```python
from build123d import *

# Parameters (mm, degrees)
SKETCH001_W     = 178
SKETCH001_H     = 55
SKETCH001_R     = 2.5
SKETCH001_R_2   = 8
SKETCH001_R_3   = 12.004096
PAD_DEPTH       = 1
SKETCH004_R     = 1.3
POCKET_DEPTH    = 9
SKETCH003_R     = 4
PAD001_DEPTH    = 8
SKETCH006_W     = 178
SKETCH006_H     = 55
SKETCH006_R     = 2.5
SKETCH006_R_2   = 8
SKETCH006_R_3   = 12.004096
PAD002_DEPTH    = 4
SKETCH_R        = 1.3
POCKET001_DEPTH = 13.001
SKETCH007_R     = 1.3
POCKET002_DEPTH = 5.001
FILLET_R        = 2


with BuildPart() as part:
    # Sketch001 → Pad (new body)
    with BuildSketch(Plane.XY):
        with Locations((-27.95005, 210.084131)):
            Rectangle(SKETCH001_W, SKETCH001_H)
        with Locations((5.54995, 200.560838)):
            Circle(SKETCH001_R, mode=Mode.SUBTRACT)
        with Locations((-105.249172, 192.692063)):
            Circle(SKETCH001_R_2, mode=Mode.SUBTRACT)
        with Locations((44.750828, 192.692063)):
            Circle(SKETCH001_R_2, mode=Mode.SUBTRACT)
        with Locations((42.270485, 220.407623)):
            Circle(SKETCH001_R_3, mode=Mode.SUBTRACT)
        with BuildLine():
            ThreePointArc((25.54995, 206.028969), (20.061493, 220.835101), (5.54995, 227.060838))
            Line((-1.19441, 227.060838), (5.54995, 227.060838))
            Line((-9.694456, 218.560838), (-1.19441, 227.060838))
            Line((-113.95005, 218.561117), (-9.694456, 218.560838))
            Line((-113.95005, 218.561117), (-113.95005, 209.560838))
            Line((-113.95005, 209.560838), (-9.618024, 209.560838))
            Line((-9.618024, 209.560838), (5.54995, 209.560838))
            Line((5.54995, 209.560838), (10.697892, 204.412896))
            Line((10.697892, 189.560838), (10.697892, 204.412896))
            ThreePointArc((10.697892, 189.560838), (21.441031, 194.803313), (25.54995, 206.028969))
        make_face(mode=Mode.SUBTRACT)
        with BuildLine():
            ThreePointArc((-74.793427, 198.14003), (-81.282837, 191.65062), (-74.793427, 185.16121))
            Line((-74.793427, 185.16121), (-26.440948, 185.16121))
            ThreePointArc((-26.440948, 185.16121), (-19.951538, 191.65062), (-26.440948, 198.14003))
            Line((-74.793427, 198.14003), (-26.440948, 198.14003))
        make_face(mode=Mode.SUBTRACT)
        with BuildLine():
            ThreePointArc((-94.612823, 233.364261), (-96.6561, 231.320984), (-94.612823, 229.277707))
            Line((-94.612823, 229.277707), (25.728859, 229.277707))
            ThreePointArc((25.728859, 229.277707), (27.772136, 231.320984), (25.728859, 233.364261))
            Line((-94.612823, 233.364261), (25.728859, 233.364261))
        make_face(mode=Mode.SUBTRACT)
    extrude(amount=PAD_DEPTH)

    # Sketch004 → Pocket (cut)
    with BuildSketch(Plane.XY.offset(10)):
        with Locations((-84.917816, 197.526398)):
            Circle(SKETCH004_R)
        with Locations((-104.937256, 231.505722)):
            Circle(SKETCH004_R)
    extrude(amount=-POCKET_DEPTH, mode=Mode.SUBTRACT)

    # Sketch003 (on Face28 of Pad) → Pad001 (join)
    with BuildSketch(Plane.XY.offset(1)):
        with Locations((-84.943253, 198.501221)):
            Circle(SKETCH003_R)
        with Locations((-104.954079, 231.041534)):
            Circle(SKETCH003_R)
    extrude(amount=PAD001_DEPTH)

    # Sketch006 → Pad002 (join)
    with BuildSketch(Plane.XY):
        with Locations((-27.95005, 210.084131)):
            Rectangle(SKETCH006_W, SKETCH006_H)
        with Locations((5.54995, 200.560838)):
            Circle(SKETCH006_R, mode=Mode.SUBTRACT)
        with Locations((-105.249172, 192.692063)):
            Circle(SKETCH006_R_2, mode=Mode.SUBTRACT)
        with Locations((44.750828, 192.692063)):
            Circle(SKETCH006_R_2, mode=Mode.SUBTRACT)
        with Locations((42.270485, 220.407623)):
            Circle(SKETCH006_R_3, mode=Mode.SUBTRACT)
        with BuildLine():
            ThreePointArc((-74.793427, 198.14003), (-81.282837, 191.65062), (-74.793427, 185.16121))
            Line((-74.793427, 185.16121), (-26.440948, 185.16121))
            ThreePointArc((-26.440948, 185.16121), (-19.951538, 191.65062), (-26.440948, 198.14003))
            Line((-74.793427, 198.14003), (-26.440948, 198.14003))
        make_face(mode=Mode.SUBTRACT)
        with BuildLine():
            ThreePointArc((-94.612823, 233.364261), (-96.6561, 231.320984), (-94.612823, 229.277707))
            Line((-94.612823, 229.277707), (25.728859, 229.277707))
            ThreePointArc((25.728859, 229.277707), (27.772136, 231.320984), (25.728859, 233.364261))
            Line((-94.612823, 233.364261), (25.728859, 233.364261))
        make_face(mode=Mode.SUBTRACT)
    extrude(amount=-PAD002_DEPTH)

    # Sketch (on Face48 of Pad002) → Pocket001 (cut, through all)
    with BuildSketch(Plane.XY.offset(9)):
        with Locations((-84.945648, 198.486725)):
            Circle(SKETCH_R)
        with Locations((-104.952744, 231.032135)):
            Circle(SKETCH_R)
    extrude(amount=-POCKET001_DEPTH, mode=Mode.SUBTRACT)

    # Sketch007 → Pocket002 (cut, through all)
    with BuildSketch(Plane.XY.offset(1)):
        with Locations((44.774215, 204.16173)):
            Circle(SKETCH007_R)
        with Locations((34.814923, 186.91173)):
            Circle(SKETCH007_R)
        with Locations((54.733507, 186.91173)):
            Circle(SKETCH007_R)
        with Locations((-107.25934, 203.941744)):
            Circle(SKETCH007_R)
        with Locations((-114.071897, 185.224398)):
            Circle(SKETCH007_R)
        with Locations((-94.455921, 188.683224)):
            Circle(SKETCH007_R)
    extrude(amount=-POCKET002_DEPTH, mode=Mode.SUBTRACT)

    # Fillet
    fillet_edges = [part.edges().sort_by_distance(p)[0] for p in [
        (-116.95005, 237.584131, -2),
        (-116.95005, 237.584131, 0.5),
        (61.04995, 237.584131, -2),
        (61.04995, 237.584131, 0.5),
        (61.04995, 182.584131, -2),
        (61.04995, 182.584131, 0.5),
        (-116.95005, 182.584131, -2),
        (-116.95005, 182.584131, 0.5),
    ]]
    fillet(fillet_edges, radius=FILLET_R)


solid = part.part
```
Geometry check sheet. Reference: the model listing, model coordinates, mm. A direction names the side the tool comes from. Round coordinates to 2 decimals unless told otherwise and drop trailing zeros. Order: outer loops, then holes, each group sorted by start corner. A loop starts at its lowest first (then second) coordinate and runs counter-clockwise, first axis right, second up. Notation, with made-up numbers: (-33.75, 30) - (14.25, 30) arc R17 cw to (14.25, 36) - close; hole circle Ø5 at (-26.75, -11). An arc over 180 degrees is marked (long way). Use a Markdown table: item, result. Add a question column.
1) Gauge pin test, flat ends, axial feed: P1, Ø3, axis at y = 199.5, z = 3.5, coming from the -X side; P2, Ø4, axis at x = -84.95, y = 198.49, coming from the -Z side; P3, Ø1, axis at y = 200, z = 2.5, coming from the +X side; P4, Ø8, axis at x = -72, y = 226, coming from the +Z side. Record the tip position at first contact, or that the pin passes through.
2) Set-up check for faces 4 (the flat face through (-29, 210, -4)), 5 (the cylindrical face through (-85.81, 194.596, 4.944)): record each of +Z, -Z, +X, -X, +Y, -Y from which the full face is reachable in a straight line by a thin tool's end or side.
3) Section check B-B (y = 217). Record the cut outline in (x, z), then the cut area to 3 significant figures.
4) Section check A-A (x = -4). Record the cut outline in (y, z).
5) Section check D-D (z = -2.5). Count the separate pieces of the cut face and the enclosed holes in it, then the cut area to 3 significant figures.
6) Mould release check, pull along X, two halves, no side actions. Record for faces 1 (the flat face through (61.05, 210, -1)), 2 (the cylindrical face through (20.217, 220.67, 0.493)), 3 (the flat face through (-29, 204, 1)): released by +X, released by -X, zero draft, split by the parting line, or undercut.
7) Section check C-C (z = 6). Record the cut outline in (x, y), then the cut area to 3 significant figures.
8) Thickness scan on line 1 along Y through (x, z) = (-86.5, 0.5); line 2 along Y through (x, z) = (18, -1.5); line 3 along Y through (x, z) = (-38, -3.5). Record the ranges inside material, lowest first.
Established:
| question | item | result |
|---|---|---|
| 1 | P1 | x = -88.94 |
| 1 | P2 | z = -4 |
| 1 | P3 | x = -81.07 |
| 1 | P4 | z = 1 |
| 2 | face 4 | -Z, +X, -X, +Y, -Y |
| 2 | face 5 | +Z |
| 3 | outline | (-116.95, -4) - (30.76, -4) - (30.76, 1) - (22.92, 1) - (22.92, 0) - (-113.95, 0) - (-113.95, 1) - (-116.95, 1) - close; (53.78, -4) - (61.05, -4) - (61.05, 1) - (53.78, 1) - close |
| 3 | area | 638 mm2 |
| 4 | outline | (182.58, -4) - (229.28, -4) - (229.28, 1) - (224.26, 1) - (224.26, 0) - (209.56, 0) - (209.56, 1) - (182.58, 1) - close; (233.36, -4) - (237.58, -4) - (237.58, 1) - (233.36, 1) - close |
| 5 | separate pieces | 1 |
| 5 | enclosed holes | 14 |
| 5 | area | 7,600 mm2 |
| 6 | face 1 | released by +X |
| 6 | face 2 | undercut |
| 6 | face 3 | zero draft |
| 7 | outline | circle Ø8 at (-104.95, 231.04); circle Ø8 at (-84.94, 198.5); hole circle Ø2.6 at (-104.95, 231.03); hole circle Ø2.6 at (-84.95, 198.49) |
| 7 | area | 89.9 mm2 |
| 8 | line 1 | 182.58 to 209.56, 218.56 to 229.28, 233.36 to 237.58 |
| 8 | line 2 | 182.58 to 229.28, 233.36 to 237.58 |
| 8 | line 3 | 182.58 to 185.16, 198.14 to 229.28, 233.36 to 237.58 |
